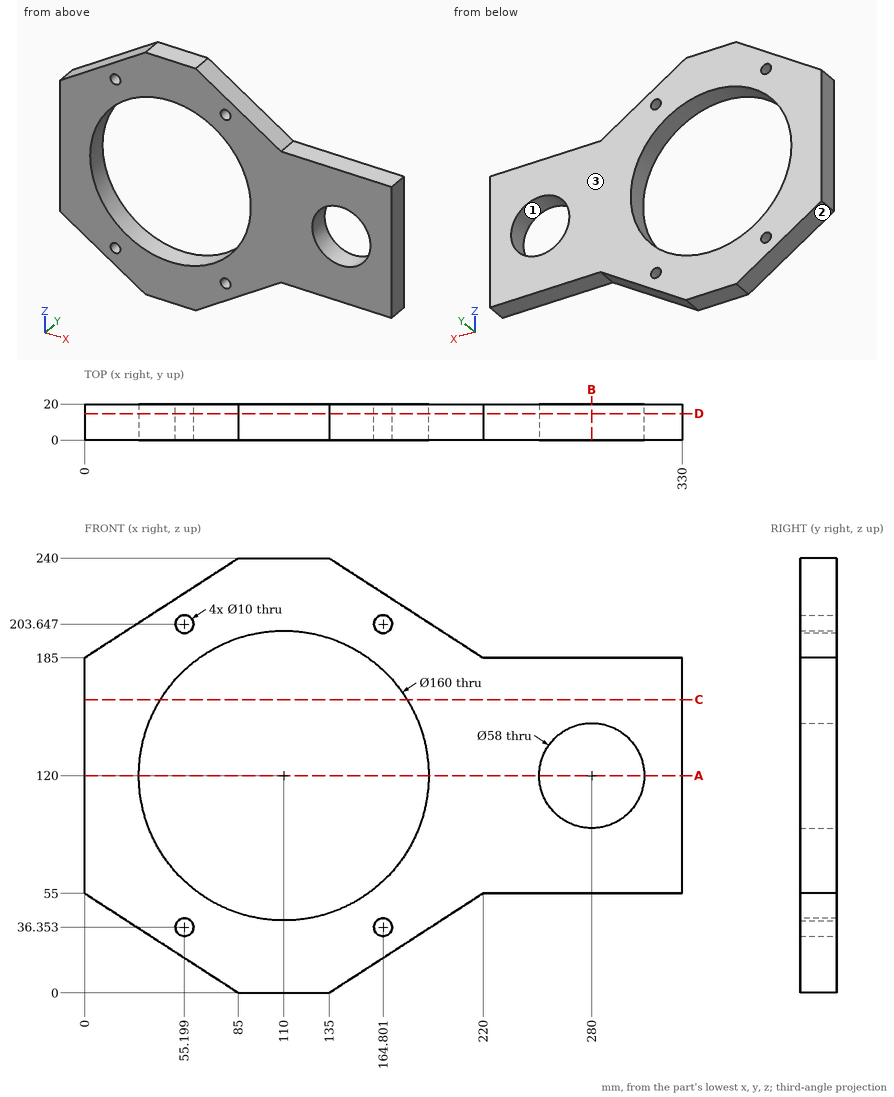
Can you work these out from the drawing? Everything is in mm from the part's minimum corner. Give positions to 0.01 mm unless a question says otherwise; leave off trailing zeros. Loops run counter-clockwise (first coordinate to the right, second up) from the corner with the lowest first, then second, coordinate; pieces in that order, holes last. Notation, with made-up numbers: (82, 28.5) -> (106, 28.5) arc R8 ccw to (106, 32.5) -> close; hole circle Ø5 at (58, 21). An arc over 180 degrees is marked (long way). Write item = value, one per line.
1) Will these pins go through, and if not, where does the flat tip stop? pin 1 (3 mm diameter, centred on y = 5.5, z = 188.5, fed in from +X); pin 2 (1.5 mm diameter, centred on y = 3.5, z = 198.5, fed in from -X) (1 decimal); pin 3 (6 mm diameter, centred on x = 213.5, y = 12, fed in from +Z).
Check result:
pin_1 = 216.91
pin_2 = 19.7
pin_3 = 191.15
2) Suppose I cut it at C-C on z = 162. Write out the boundary of the cut face in (x, y).
Check result:
outline = (0, 0) -> (41.91, 0) -> (41.91, 20) -> (0, 20) -> close; (178.09, 0) -> (330, 0) -> (330, 20) -> (178.09, 20) -> close
3) Suppose I cut it at D-D on y = 14.75. Write out the boundary of the cut face in (x, z).
Check result:
outline = (0, 55) -> (85, 0) -> (135, 0) -> (220, 55) -> (330, 55) -> (330, 185) -> (220, 185) -> (135, 240) -> (85, 240) -> (0, 185) -> close; hole circle Ø160 at (110, 120); hole circle Ø10 at (55.2, 36.35); hole circle Ø10 at (55.2, 203.65); hole circle Ø10 at (164.8, 36.35); hole circle Ø10 at (164.8, 203.65); hole circle Ø58 at (280, 120)
4) Thinking about a two-plate mould opening in Z: for the marked faces 1, 2 and 3, which applies, released by +Z, released by -Z, zero draft, split by the parting line, or undercut?
Check result:
face_1 = undercut
face_2 = released by -Z
face_3 = zero draft
5) Suppose I cut it at A-A on z = 120. Write out the boundary of the cut face in (x, y), then the cut area to 3 significant figures.
Check result:
outline = (0, 0) -> (30, 0) -> (30, 20) -> (0, 20) -> close; (190, 0) -> (251, 0) -> (251, 20) -> (190, 20) -> close; (309, 0) -> (330, 0) -> (330, 20) -> (309, 20) -> close
area = 2,240 mm2
6) I need wall thicknesses on L1, parallel to Z at x = 280, y = 13.5; L2, parallel to Z at x = 311, y = 5; L3, parallel to X at y = 19.25, z = 94.5. Which ranges of each line are inside material? Lowest first, please. Write a range as from..to.
Check result:
L1 = 55..91, 149..185
L2 = 55..185
L3 = 0..34.17, 185.83..266.19, 293.81..330
7) Suppose I cut it at B-B on x = 280. Write out the boundary of the cut face in (y, z), then the cut area to 3 significant figures.
Check result:
outline = (0, 55) -> (20, 55) -> (20, 91) -> (0, 91) -> close; (0, 149) -> (20, 149) -> (20, 185) -> (0, 185) -> close
area = 1,440 mm2
